Here's how the part is built. I have some questions about the finished solid (model axes, mm). A direction names the side the tool comes from. Give positions to 0.01 mm unless a question says otherwise; leave off trailing zeros. Loops run counter-clockwise (first coordinate to the right, second up) from the corner with the lowest first, then second, coordinate; pieces in that order, holes last. Notation, with made-up numbers: (61.25, 1.5) - (66.25, 1.5) arc R20 ccw to (66.25, 5.5) - close; hole circle Ø9 at (-5.75, 58). An arc over 180 degrees is marked (long way). Use one line per item in the form item = value.
from build123d import *

# Parameters (mm, degrees)
F1_DEPTH = 9.525
F2_SIZE  = 1.27


with BuildPart() as f1:
    # F0 (on Top) → F1 (new body)
    with BuildSketch(Plane.XY):
        with BuildLine():
            ThreePointArc((33.019756, -0.127), (-33.02, 0), (33.019756, 0.126999))
            Line((33.019756, 0.126999), (42.54481, 0.126999))
            ThreePointArc((42.54481, 0.126999), (-42.545, 0), (42.54481, -0.126999))
            Line((42.54481, -0.126999), (33.019756, -0.127))
        make_face()
    extrude(amount=F1_DEPTH)

    # F2
    f2_edges = [f1.edges().sort_by_distance(p)[0] for p in [
        (-42.545, 0, 9.525),
        (-42.545, 0, 0),
        (-33.02, 0, 9.525),
        (-33.02, 0, 0),
    ]]
    chamfer(f2_edges, length=F2_SIZE)


solid = f1.part
(1) For P1, Ø1, axis at x = 1, z = 5.5, coming from the -Y side; P2, Ø2, axis at x = 33.5, z = 4.5, coming from the +Y side; P3, Ø3, axis at x = 36, z = 2.5, coming from the -Y side, each with a flat end and sliding along its axis, tell me the tip position at first contact or that it passes through.
Geometry says:
P1 = -42.54
P2 = 27.46
P3 = -24.9
(2) If we section it at A-A (x = 0): List the corners of the cut face in (y, z) for me (3 decimals).
Geometry says:
outline = (-42.545, 1.27) - (-41.275, 0) - (-34.29, 0) - (-33.02, 1.27) - (-33.02, 8.255) - (-34.29, 9.525) - (-41.275, 9.525) - (-42.545, 8.255) - close; (33.02, 1.27) - (34.29, 0) - (41.275, 0) - (42.545, 1.27) - (42.545, 8.255) - (41.275, 9.525) - (34.29, 9.525) - (33.02, 8.255) - close
(3) If we section it at B-B (z = 3.5): List the corners of the cut face in (x, y) for me (3 decimals), plus the area to 3 significant figures.
Geometry says:
outline = (33.02, -0.127) arc R33.02 cw (long way) to (33.02, 0.127) - (42.545, 0.127) arc R42.545 ccw (long way) to (42.545, -0.127) - close
area = 2,260 mm²
(4) If I drill on probe 1 along Y at (x, z) = (0, 4.5) (3 decimals); probe 2 along X at (y, z) = (0, 5) (3 decimals); probe 3 along Y at (x, z) = (-13, 1), over which ranges is the centre line in solid material (lowest first)?
Geometry says:
probe_1 = -42.545 to -33.02, 33.02 to 42.545
probe_2 = -42.545 to -33.02
probe_3 = -40.23 to -30.65, 30.65 to 40.23
(5) For faces 1 (the flat face through (38, -0.127, 5)), 2 (the flat face through (6, 34, 9.525)), which set-ups out of +Z, -Z, +X, -X, +Y, -Y let a thin tool reach every point of the face, with its end or its side?
Geometry says:
face_1 = +Z, -Z, +X
face_2 = +Z, +X, -X, +Y, -Y
(6) Thinking about a two-plate mould opening in Y: for faces 3 (the flat face through (38, 0.127, 5)), 4 (the flat face through (6, 34, 0)), 5 (the cylindrical face through (-42.504, 1.869, 4.714)), which applies, pulls with the +Y half, pulls with the -Y half, needs draft (parallel to the pull), parting line crosses it, or undercut?
Geometry says:
face_3 = undercut
face_4 = needs draft
face_5 = parting line crosses it
